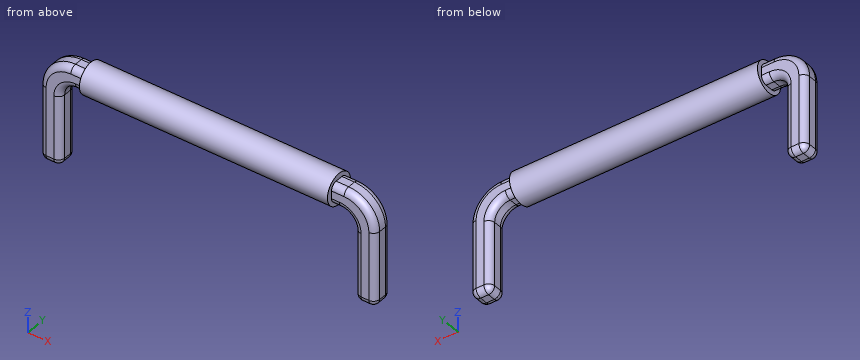
Autodesk Fusion 360 part; units mm, degrees
sketch "Sketch1" plane through (0, 0, 0) normal (1, 0, 0) x (0, 1, 0)
  circle A0 centre (0, 0) radius 0.5
  line L0 (0.325, -0.325) -> (-0.325, -0.325)
  line L1 (-0.325, -0.325) -> (-0.325, 0.325)
  line L2 (-0.325, 0.325) -> (0.325, 0.325)
  line L3 (0.325, 0.325) -> (0.325, -0.325)
  line L4 (0.325, -0.325) -> (-0.325, 0.325) construction
  line L5 (-0.325, -0.325) -> (0.325, 0.325) construction
  dimension "d1" = 1
  dimension "d2" = 0.65
  dimension "d3" = 0.65
extrude "Extrude1" add sketch "Sketch1" along normal blind 8 contours A0 | L0 L1 L2 L3
sketch "Sketch2" plane through (8, 0, 0) normal (1, 0, 0) x (0, 1, 0)
  circle A0 centre (0, 0) radius 0.5
  line L0 (0.325, -0.325) -> (-0.325, -0.325)
  line L1 (-0.325, -0.325) -> (-0.325, 0.325)
  line L2 (-0.325, 0.325) -> (0.325, 0.325)
  line L3 (0.325, 0.325) -> (0.325, -0.325)
  line L4 (0.325, -0.325) -> (-0.325, 0.325) construction
  line L5 (-0.325, -0.325) -> (0.325, 0.325) construction
  dimension "d8" = 0.65
  dimension "d9" = 0.65
extrude "Extrude2" add sketch "Sketch2" along normal blind 1.405 contours L0 L1 L2 L3
extrude "Extrude3" add sketch "Sketch1" against normal blind 1.405 contours L0 L1 L2 L3
sketch "Sketch3" plane through (0, 0, -0.325) normal (0, 0, -1) x (1, 0, 0)
  line L0 (8, 0.325) -> (8, -0.325)
  line L1 (8, -0.325) -> (9.405, -0.325)
  line L2 (9.405, -0.325) -> (9.405, 0.325)
  line L3 (9.405, 0.325) -> (8, 0.325)
  line L4 (9.405, 0.325) -> (8.755, 0.325)
  line L5 (8.755, 0.325) -> (8.755, -0.325)
  line L6 (8.755, -0.325) -> (9.405, -0.325)
  line L7 (9.405, -0.325) -> (9.405, 0.325)
  line L8 (9.405, 0.325) -> (8.755, -0.325) construction
  line L9 (8.755, 0.325) -> (9.405, -0.325) construction
  point P0 (9.08, 0)
  dimension "d14" = 0.65
  dimension "d15" = 0.65
sketch "Sketch4" plane through (0, 0, -0.325) normal (0, 0, -1) x (1, 0, 0)
  line L0 (0, -0.325) -> (0, 0.325)
  line L1 (0, 0.325) -> (-1.405, 0.325)
  line L2 (-1.405, 0.325) -> (-1.405, -0.325)
  line L3 (-1.405, -0.325) -> (0, -0.325)
  line L4 (-0.755, -0.325) -> (-1.405, -0.325)
  line L5 (-1.405, -0.325) -> (-1.405, 0.325)
  line L6 (-1.405, 0.325) -> (-0.755, 0.325)
  line L7 (-0.755, 0.325) -> (-0.755, -0.325)
  line L8 (-0.755, -0.325) -> (-1.405, 0.325) construction
  line L9 (-1.405, -0.325) -> (-0.755, 0.325) construction
  point P0 (-1.08, 0)
  dimension "d17" = 0.65
  dimension "d18" = 0.65
extrude "Extrude4" add sketch "Sketch4" sketch "Sketch3" along normal blind 2.75 contours L1 L2 L3 L4 L5 L6 L7 of sketch 2 contours L1 L2 L3 L4 L5 L6 L7
fillet "Fillet1" radius 0.5 2 edges at (-0.755, 0, -0.325) (8.755, 0, -0.325)
fillet "Fillet2" radius 1 2 edges at (-1.405, 0, 0.325) (9.405, 0, 0.325)
fillet "Fillet3" radius 0.2 28 edges at (-1.08, -0.325, -3.075) (-0.755, 0, -3.075) (-1.08, 0.325, -3.075) (-1.405, 0, -3.075) (-0.6086, -0.325, -0.4714) (-0.755, -0.325, -1.95) (-0.2025, -0.325, 0.325) (-1.1121, -0.325, 0.0321) (-1.405, -0.325, -1.875) (-0.2025, 0.325, 0.325) (-1.1121, 0.325, 0.0321) (-1.405, 0.325, -1.875) (-0.6086, 0.325, -0.4714) (-0.755, 0.325, -1.95) (8.2025, -0.325, 0.325) (9.1121, -0.325, 0.0321) (9.405, -0.325, -1.875) (8.755, -0.325, -1.95) (8.6086, -0.325, -0.4714) (9.405, 0.325, -1.875) (9.1121, 0.325, 0.0321) (8.2025, 0.325, 0.325) (8.6086, 0.325, -0.4714) (8.755, 0.325, -1.95) (9.08, 0.325, -3.075) (9.405, 0, -3.075) (9.08, -0.325, -3.075) (8.755, 0, -3.075)
equation "d1 = width"
equation "d2 = d3"
equation "d3 = d1 * 0.65"
equation "width = 1 mm"
equation "baseLenght = 8 mm"
equation "d6 = baseLenght"
equation "d8 = width * 0.65"
equation "d9 = d8"
equation "d14 = width * 0.65"
equation "d15 = d14"
equation "d17 = width * 0.65"
equation "d18 = d17"
equation "d26 = 0.2 * width"
Can you work these out from the model? Positions are in its coordinate system, mm. Give positions to 0.01 mm unless a question says otherwise; leave off trailing zeros. Write each loop counter-clockwise with the first axis right and the second up, starting at its lowest first coordinate (ties: lowest second). Pieces come first, ordered by that corner, then holes. Notation, with made-up numbers: (-10, -5.5) - (44, -5.5) arc R23 ccw to (44, 29.5) - close; hole circle Ø5 at (36, 17.5). An arc over 180 degrees is marked (long way). Write item = value, one per line. Start each with the question number.
1. For pin 1 (1 mm diameter, centred on x = 8.5, z = -1.5, fed in from +Y) (3 decimals); pin 2 (1.5 mm diameter, centred on x = 2.5, z = -2.5, fed in from -Y); pin 3 (0.6 mm diameter, centred on x = 9, z = -1.5, fed in from -Y) (3 decimals); pin 4 (0.5 mm diameter, centred on y = 0, z = 0, fed in from -X), each with a flat end and sliding along its axis, tell me the tip position at first contact or that it passes through.
2. Please list where these lines run through material, in increasing order: line 1 (X direction, y = -0.05, z = -2.55) (3 decimals); line 2 (X direction, y = -0.4, z = -0.15); line 3 (Z direction, x = 6.5, y = 0).
3. Imagine slicing it at B-B (y = 0). Please give me the cut outline in (x, z) (3 decimals).
4. Imagine slicing it at C-C (x = 2.5). Please give me the cut outline in (y, z).
5. Imagine slicing it at A-A (z = -1.7). Please give me the cut outline in (x, y) (3 decimals), and give its area (3 significant figures).
Worked answers:
q1.pin_1 = 0.325
q1.pin_2 = through
q1.pin_3 = -0.325
q1.pin_4 = -1.31
q2.line_1 = -1.405 to -0.755, 8.755 to 9.405
q2.line_2 = 0 to 8
q2.line_3 = -0.5 to 0.5
q3.outline = (-1.405, -2.875) arc R0.2 ccw to (-1.205, -3.075) - (-0.955, -3.075) arc R0.2 ccw to (-0.755, -2.875) - (-0.755, -0.825) arc R0.5 cw to (-0.255, -0.325) - (0, -0.325) - (0, -0.5) - (8, -0.5) - (8, -0.325) - (8.255, -0.325) arc R0.5 cw to (8.755, -0.825) - (8.755, -2.875) arc R0.2 ccw to (8.955, -3.075) - (9.205, -3.075) arc R0.2 ccw to (9.405, -2.875) - (9.405, -0.675) arc R1 ccw to (8.405, 0.325) - (8, 0.325) - (8, 0.5) - (0, 0.5) - (0, 0.325) - (-0.405, 0.325) arc R1 ccw to (-1.405, -0.675) - close
q4.outline = circle Ø1 at (0, 0)
q5.outline = (-1.405, -0.125) arc R0.2 ccw to (-1.205, -0.325) - (-0.955, -0.325) arc R0.2 ccw to (-0.755, -0.125) - (-0.755, 0.125) arc R0.2 ccw to (-0.955, 0.325) - (-1.205, 0.325) arc R0.2 ccw to (-1.405, 0.125) - close; (8.755, -0.125) arc R0.2 ccw to (8.955, -0.325) - (9.205, -0.325) arc R0.2 ccw to (9.405, -0.125) - (9.405, 0.125) arc R0.2 ccw to (9.205, 0.325) - (8.955, 0.325) arc R0.2 ccw to (8.755, 0.125) - close
q5.area = 0.776 mm2
